The model under review builds one solid part; all positions refer to its coordinate system, in mm. Face numbers are marked on the shaded views. Give positions to 0.01 mm unless a question says otherwise; leave off trailing zeros. Loops run counter-clockwise (first coordinate to the right, second up) from the corner with the lowest first, then second, coordinate; pieces in that order, holes last. Notation, with made-up numbers: M -16,37.5 L 3,37.5 A9 cw 3,50.5 Z; hole C -25,8 d1. An arc over 180 degrees is marked long. Return JSON: item names as keys, results as strings.
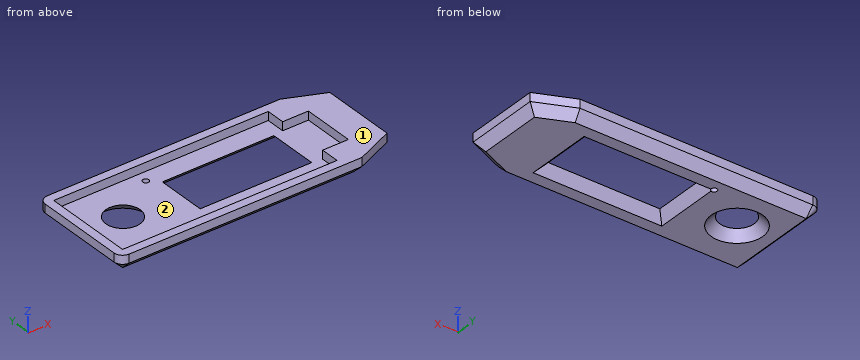
```python
from build123d import *

# Parameters (mm, degrees)
EXTRUDE_1_DEPTH     = 2
EXTRUDE_2_DEPTH     = 2
SKETCH_4_R          = 4
SKETCH_4_R_2        = 0.7
SKETCH_4_W          = 26
SKETCH_4_H          = 11.55
CUT_EXTRUDE_1_DEPTH = 49.322997027
CHAMFER_3_SIZE      = 2
FILLET_2_R          = 2
CHAMFER_4_SIZE      = 2


# Some blends are built 0.0001 mm under size
with BuildPart() as part:
    # Эскиз1 → Бобышка-Вытянуть1 (new body)
    with BuildSketch(Plane.XY):
        Polygon((46.296875, 9.92578125), (37.5703125, 13.70078125), (-18.703125, 13.70078125), (-18.703125, -11.29921875), (37.5703125, -11.29921875), (46.296875, -7.52421875), align=None)
    extrude(amount=EXTRUDE_1_DEPTH)

    # Эскиз2 → Бобышка-Вытянуть2 (add)
    with BuildSketch(Plane.XY.offset(2)):
        Polygon((-18.703125, -11.29921875), (37.5703125, -11.29921875), (46.296875, -7.52421875), (46.296875, 9.92578125), (37.5703125, 13.70078125), (-18.703125, 13.70078125), align=None)
        Polygon((-16.703125, 11.70078125), (33.296875, 11.70078125), (33.296875, 7.30078125), (39.296875, 7.30078125), (39.296875, -4.89921875), (33.296875, -4.89921875), (33.296875, -9.29921875), (-16.703125, -9.29921875), align=None, mode=Mode.SUBTRACT)
    extrude(amount=EXTRUDE_2_DEPTH)

    # Эскиз4 → Вырез-Вытянуть1 (cut, through all)
    with BuildSketch(Plane.XY.offset(2)):
        with Locations((-8.003125, 1.96785345)):
            Circle(SKETCH_4_R)
        with Locations((2.756875, 9.10078125)):
            Circle(SKETCH_4_R_2)
        with Locations((17.996875, 1.20078125)):
            Rectangle(SKETCH_4_W, SKETCH_4_H)
    extrude(amount=-CUT_EXTRUDE_1_DEPTH, mode=Mode.SUBTRACT)

    # Фаска3
    # the kernel refuses this chamfer: 2 mm, written as the material it takes off along each edge
    with BuildSketch(Plane(origin=(51.017483297, 7.883706112, 0), x_dir=(0.010916712185249174, 0.025235859914990173, 0.9996219169112968), z_dir=(-0.9178052503070296, 0.3970308835705994, 0))) as chamfer_3_piece_1:
        Polygon((CHAMFER_3_SIZE * 0.999621916911, -CHAMFER_3_SIZE * 0.0274958766106), (-CHAMFER_3_SIZE * 0.0274958766106, -CHAMFER_3_SIZE * 0.999621916911), (0, 0), align=None)
    extrude(amount=19.794808417, mode=Mode.SUBTRACT)
    with BuildSketch(Plane(origin=(46.296875, -12.667584726, 0), x_dir=(0.02749587661058563, 0, 0.9996219169112968), z_dir=(0, 1, 0))) as chamfer_3_piece_2:
        Polygon((CHAMFER_3_SIZE * 0.999621916911, -CHAMFER_3_SIZE * 0.0274958766106), (-CHAMFER_3_SIZE * 0.0274958766106, -CHAMFER_3_SIZE * 0.999621916911), (0, 0), align=None)
    extrude(amount=27.736731952, mode=Mode.SUBTRACT)
    with BuildSketch(Plane(origin=(32.849704203, -13.341293888, 0), x_dir=(-0.3968807729078274, 0.9174582436631658, -0.027495876610586396), z_dir=(0.91780525030703, 0.3970308835705984, 0))) as chamfer_3_piece_3:
        Polygon((CHAMFER_3_SIZE * 0.999621916911, CHAMFER_3_SIZE * 0.0274958766106), (-CHAMFER_3_SIZE * 0.0274958766106, CHAMFER_3_SIZE * 0.999621916911), (0, 0), align=None)
    extrude(amount=19.794808417, mode=Mode.SUBTRACT)
    with BuildSketch(Plane(origin=(-8.003125, 1.96785345, 0), x_dir=(1, 0, 0), z_dir=(0, -1, 0))) as chamfer_3_piece_4:
        Polygon((4 + CHAMFER_3_SIZE, 0), (4, CHAMFER_3_SIZE), (4, 0), align=None)
    revolve(axis=Axis((-8.003125, 1.96785345, 0), (0, 0, 1)), mode=Mode.SUBTRACT)
    with BuildSketch(Plane(origin=(30.996875, 6.97578125, 0), x_dir=(0.9996219169112968, 0, -0.02749587661058632), z_dir=(0, -1, 0)), Plane(origin=(4.996875, -4.57421875, 0), x_dir=(-0.9996219169112968, 0, -0.027495876610586372), z_dir=(0, 1, 0))) as chamfer_3_piece_5:
        Polygon((CHAMFER_3_SIZE * 0.999621916911, CHAMFER_3_SIZE * 0.0274958766106), (-CHAMFER_3_SIZE * 0.0274958766106, CHAMFER_3_SIZE * 0.999621916911), (0, 0), align=None)
    extrude(amount=11.55, mode=Mode.SUBTRACT)
    with BuildSketch(Plane(origin=(30.996875, -4.57421875, 0), x_dir=(0, -0.9996219169112968, -0.027495876610586365), z_dir=(-1, 0, 0)), Plane(origin=(4.996875, 6.97578125, 0), x_dir=(0, 0.9996219169112968, -0.027495876610586348), z_dir=(1, 0, 0))) as chamfer_3_piece_6:
        Polygon((CHAMFER_3_SIZE * 0.999621916911, CHAMFER_3_SIZE * 0.0274958766106), (-CHAMFER_3_SIZE * 0.0274958766106, CHAMFER_3_SIZE * 0.999621916911), (0, 0), align=None)
    extrude(amount=26, mode=Mode.SUBTRACT)
    with BuildSketch(Plane(origin=(30.996875, 12.119147226, 0), x_dir=(0.9996219169112968, 0, -0.02749587661058632), z_dir=(0, -1, 0))) as chamfer_3_piece_7a_section:
        Polygon((CHAMFER_3_SIZE * 0.999621916911, CHAMFER_3_SIZE * 0.0274958766106), (-CHAMFER_3_SIZE * 0.0274958766106, CHAMFER_3_SIZE * 0.999621916911), (0, 0), align=None)
    chamfer_3_piece_7a = extrude(amount=16.693365976, mode=Mode.PRIVATE)
    chamfer_3_piece_7a = split(chamfer_3_piece_7a, bisect_by=Plane(origin=(31.656462254, 6.97578125, 0.659587254), z_dir=(0, 1, 0)), keep=Keep.TOP, mode=Mode.PRIVATE)
    with BuildSketch(Plane(origin=(4.996875, 6.97578125, 0), x_dir=(0, 0.9996219169112968, -0.027495876610586348), z_dir=(1, 0, 0))) as chamfer_3_piece_7b_section:
        Polygon((CHAMFER_3_SIZE * 0.999621916911, CHAMFER_3_SIZE * 0.0274958766106), (-CHAMFER_3_SIZE * 0.0274958766106, CHAMFER_3_SIZE * 0.999621916911), (0, 0), align=None)
    chamfer_3_piece_7b = extrude(amount=31.143365976, mode=Mode.PRIVATE)
    chamfer_3_piece_7b = split(chamfer_3_piece_7b, bisect_by=Plane(origin=(30.996875, 7.635368504, 0.659587254), z_dir=(1, 0, 0)), keep=Keep.TOP, mode=Mode.PRIVATE)
    chamfer_3_piece_7 = chamfer_3_piece_7a & chamfer_3_piece_7b
    add(chamfer_3_piece_7, mode=Mode.SUBTRACT)
    with BuildSketch(Plane(origin=(36.140240976, -4.57421875, 0), x_dir=(0, -0.9996219169112968, -0.027495876610586365), z_dir=(-1, 0, 0))) as chamfer_3_piece_8a_section:
        Polygon((CHAMFER_3_SIZE * 0.999621916911, CHAMFER_3_SIZE * 0.0274958766106), (-CHAMFER_3_SIZE * 0.0274958766106, CHAMFER_3_SIZE * 0.999621916911), (0, 0), align=None)
    chamfer_3_piece_8a = extrude(amount=31.143365976, mode=Mode.PRIVATE)
    chamfer_3_piece_8a = split(chamfer_3_piece_8a, bisect_by=Plane(origin=(30.996875, -5.233806004, 0.659587254), z_dir=(1, 0, 0)), keep=Keep.TOP, mode=Mode.PRIVATE)
    with BuildSketch(Plane(origin=(30.996875, 6.97578125, 0), x_dir=(0.9996219169112968, 0, -0.02749587661058632), z_dir=(0, -1, 0))) as chamfer_3_piece_8b_section:
        Polygon((CHAMFER_3_SIZE * 0.999621916911, CHAMFER_3_SIZE * 0.0274958766106), (-CHAMFER_3_SIZE * 0.0274958766106, CHAMFER_3_SIZE * 0.999621916911), (0, 0), align=None)
    chamfer_3_piece_8b = extrude(amount=16.693365976, mode=Mode.PRIVATE)
    chamfer_3_piece_8b = split(chamfer_3_piece_8b, bisect_by=Plane(origin=(31.656462254, -4.57421875, 0.659587254), z_dir=(0, -1, 0)), keep=Keep.TOP, mode=Mode.PRIVATE)
    chamfer_3_piece_8 = chamfer_3_piece_8a & chamfer_3_piece_8b
    add(chamfer_3_piece_8, mode=Mode.SUBTRACT)
    with BuildSketch(Plane(origin=(4.996875, -9.717584726, 0), x_dir=(-0.9996219169112968, 0, -0.027495876610586355), z_dir=(0, 1, 0))) as chamfer_3_piece_9a_section:
        Polygon((CHAMFER_3_SIZE * 0.999621916911, CHAMFER_3_SIZE * 0.0274958766106), (-CHAMFER_3_SIZE * 0.0274958766106, CHAMFER_3_SIZE * 0.999621916911), (0, 0), align=None)
    chamfer_3_piece_9a = extrude(amount=16.693365976, mode=Mode.PRIVATE)
    chamfer_3_piece_9a = split(chamfer_3_piece_9a, bisect_by=Plane(origin=(4.337287746, -4.57421875, 0.659587254), z_dir=(0, -1, 0)), keep=Keep.TOP, mode=Mode.PRIVATE)
    with BuildSketch(Plane(origin=(30.996875, -4.57421875, 0), x_dir=(0, -0.9996219169112968, -0.027495876610586365), z_dir=(-1, 0, 0))) as chamfer_3_piece_9b_section:
        Polygon((CHAMFER_3_SIZE * 0.999621916911, CHAMFER_3_SIZE * 0.0274958766106), (-CHAMFER_3_SIZE * 0.0274958766106, CHAMFER_3_SIZE * 0.999621916911), (0, 0), align=None)
    chamfer_3_piece_9b = extrude(amount=31.143365976, mode=Mode.PRIVATE)
    chamfer_3_piece_9b = split(chamfer_3_piece_9b, bisect_by=Plane(origin=(4.996875, -5.233806004, 0.659587254), z_dir=(-1, 0, 0)), keep=Keep.TOP, mode=Mode.PRIVATE)
    chamfer_3_piece_9 = chamfer_3_piece_9a & chamfer_3_piece_9b
    add(chamfer_3_piece_9, mode=Mode.SUBTRACT)
    with BuildSketch(Plane(origin=(4.996875, -4.57421875, 0), x_dir=(-0.9996219169112968, 0, -0.027495876610586372), z_dir=(0, 1, 0))) as chamfer_3_piece_10a_section:
        Polygon((CHAMFER_3_SIZE * 0.999621916911, CHAMFER_3_SIZE * 0.0274958766106), (-CHAMFER_3_SIZE * 0.0274958766106, CHAMFER_3_SIZE * 0.999621916911), (0, 0), align=None)
    chamfer_3_piece_10a = extrude(amount=16.693365976, mode=Mode.PRIVATE)
    chamfer_3_piece_10a = split(chamfer_3_piece_10a, bisect_by=Plane(origin=(4.337287746, 6.97578125, 0.659587254), z_dir=(0, 1, 0)), keep=Keep.TOP, mode=Mode.PRIVATE)
    with BuildSketch(Plane(origin=(-0.146490976, 6.97578125, 0), x_dir=(0, 0.9996219169112968, -0.027495876610586348), z_dir=(1, 0, 0))) as chamfer_3_piece_10b_section:
        Polygon((CHAMFER_3_SIZE * 0.999621916911, CHAMFER_3_SIZE * 0.0274958766106), (-CHAMFER_3_SIZE * 0.0274958766106, CHAMFER_3_SIZE * 0.999621916911), (0, 0), align=None)
    chamfer_3_piece_10b = extrude(amount=31.143365976, mode=Mode.PRIVATE)
    chamfer_3_piece_10b = split(chamfer_3_piece_10b, bisect_by=Plane(origin=(4.996875, 7.635368504, 0.659587254), z_dir=(-1, 0, 0)), keep=Keep.TOP, mode=Mode.PRIVATE)
    chamfer_3_piece_10 = chamfer_3_piece_10a & chamfer_3_piece_10b
    add(chamfer_3_piece_10, mode=Mode.SUBTRACT)

    # Скругление2
    fillet_2_edges = [part.edges().sort_by_distance(p)[0] for p in [
        (-18.703125, 13.70078125, 2),
        (-18.703125, -11.29921875, 2),
    ]]
    fillet(fillet_2_edges, radius=FILLET_2_R)

    # Фаска4
    chamfer_4_edges = [part.edges().sort_by_distance(p)[0] for p in [
        (7.914897998, -11.29921875, 0),
        (-18.117338562, -10.713432312, 0),
        (-18.703125, 1.20078125, 0),
        (-18.117338562, 13.114994812, 0),
        (7.914897998, 13.70078125, 0),
    ]]
    chamfer(chamfer_4_edges, length=CHAMFER_4_SIZE - 0.0001)  # a hair under: the kernel refuses the full size


solid = part.part
```
1) The part is to be moulded in two halves that separate along X. For the marked faces 1 and 2, say which applies: released by +X, released by -X, zero draft, split by the parting line, or undercut.
From the geometry:
{"face 1": "zero draft", "face 2": "undercut"}
2) Consider section C-C on x = 34.5. Write out the cut boundary in (y, z), then the cut area to 3 significant figures.
From the geometry:
{"outline": "M -11.3,2 L -9.3,0 L 11.7,0 L 13.7,2 L 13.7,4 L 7.3,4 L 7.3,2 L -4.9,2 L -4.9,4 L -11.3,4 Z", "area": "71.6 mm²"}
3) Consider section A-A on x = 27. Write out the cut boundary in (y, z).
From the geometry:
{"outline": "M -11.3,2 L -9.3,0 L -6.57,0 L -4.57,2 L -9.3,2 L -9.3,4 L -11.3,4 Z; M 6.98,2 L 8.98,0 L 11.7,0 L 13.7,2 L 13.7,4 L 11.7,4 L 11.7,2 Z"}
4) Consider section B-B on z = 2.65. Write out the cut boundary in (x, y).
From the geometry:
{"outline": "M -18.7,-9.3 A2 ccw -16.7,-11.3 L 37.57,-11.3 L 46.3,-7.52 L 46.3,9.93 L 37.57,13.7 L -16.7,13.7 A2 ccw -18.7,11.7 Z; hole M -16.7,-9.3 L 33.3,-9.3 L 33.3,-4.9 L 39.3,-4.9 L 39.3,7.3 L 33.3,7.3 L 33.3,11.7 L -16.7,11.7 Z"}
5) Insertion check: pin 1 (10.5 mm diameter, centred on x = 20.5, y = -2, fed in from +Z). The pin has a flat end and moves straight along its axis. Give the tip position at first contact, or say it passes through.
From the geometry:
{"pin 1": "z = 2"}
6) Consider section D-D on y = 4. Count the separate pieces of the cut face and the enclosed holes in it, then the cut area to 3 significant figures.
From the geometry:
{"separate pieces": "3", "enclosed holes": "0", "area": "69.8 mm²"}
7) Wall thickness on L1, parallel to X at y = 9.5, z = 2.1; L2, parallel to Y at x = -4, z = 3.5; L3, parallel to X at y = 1.5, z = 3.5: over which ranges is each line inside the solid? List them lowest first. Write a range as from..to.
From the geometry:
{"L1": "-18.7..-16.7, 33.3..46.3", "L2": "-11.3..-9.3, 11.7..13.7", "L3": "-18.7..-16.7, 39.3..46.3"}
